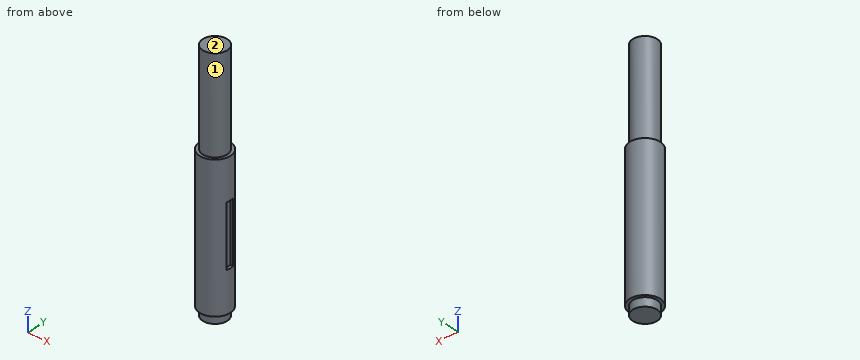
from build123d import *

# Parameters (mm, degrees)
SKETCH1_R           = 12.5
BOSS_EXTRUDE1_DEPTH = 116
SKETCH2_R           = 10
BOSS_EXTRUDE2_DEPTH = 7
BOSS_EXTRUDE3_START = 7
SKETCH3_R           = 10
BOSS_EXTRUDE3_DEPTH = 7
SKETCH4_W           = 50
SKETCH4_H           = 6.35
CUT_EXTRUDE1_DEPTH  = 2.38125
SKETCH6_R           = 10
BOSS_EXTRUDE4_DEPTH = 70


with BuildPart() as part:
    # Sketch1 → Boss-Extrude1 (new body)
    with BuildSketch(Plane.XY):
        with Locations(Location((0, 0, 0), (0, 0, 180))):
            Circle(SKETCH1_R)
    extrude(amount=BOSS_EXTRUDE1_DEPTH)

    # Sketch2 → Boss-Extrude2 (add)
    with BuildSketch(Plane.XY.offset(116)):
        Circle(SKETCH2_R)
    extrude(amount=BOSS_EXTRUDE2_DEPTH)

    # Sketch3 → Boss-Extrude3 (add)
    with BuildSketch(Plane(origin=(0, 0, 0), x_dir=(-1, 0, 0), z_dir=(0, 0, -1)).offset(BOSS_EXTRUDE3_START)):
        with Locations(Location((0, 0, 0), (0, 0, 180))):
            Circle(SKETCH3_R)
    extrude(amount=-BOSS_EXTRUDE3_DEPTH)

    # Sketch4 → Cut-Extrude1 (cut)
    with BuildSketch(Plane(origin=(12.5, 0, 0), x_dir=(0, 0, -1), z_dir=(1, 0, 0))):
        with Locations((-58, 0)):
            Rectangle(SKETCH4_W, SKETCH4_H)
    extrude(amount=-CUT_EXTRUDE1_DEPTH, mode=Mode.SUBTRACT)

    # Sketch6 → Boss-Extrude4 (add)
    with BuildSketch(Plane.XY.offset(123)):
        Circle(SKETCH6_R)
    extrude(amount=BOSS_EXTRUDE4_DEPTH)


solid = part.part
Verification items for the finished model (mm, model axes). Face numbers are marked on the shaded views. A direction names the side the tool comes from. Round coordinates to 2 decimals unless told otherwise and drop trailing zeros. Loops run counter-clockwise (first coordinate to the right, second up) from the corner with the lowest first, then second, coordinate; pieces in that order, holes last. Notation, with made-up numbers: (81, 35.25) - (105, 35.25) arc R4 cw to (105, 41.25) - close; hole circle Ø11 at (25, -6.75). An arc over 180 degrees is marked (long way). Use a Markdown table: item, result. Add a question column.
1. Section check A-A, the plane y = 0. Record the boundary of the cut face in (x, z).
2. Thickness scan on probe 1 along X at (y, z) = (-7.5, 8); probe 2 along Z at (x, y) = (-4.5, -9); probe 3 along Y at (x, z) = (0, 66.5). Record the ranges inside material, lowest first. Write a range as [from, to].
3. Gauge pin test, flat ends, axial feed: pin 1 (8 mm diameter, centred on y = 4.5, z = 102, fed in from -X); pin 2 (3 mm diameter, centred on y = -1, z = 55.5, fed in from +X); pin 3 (2 mm diameter, centred on y = -2.5, z = 31, fed in from +X). Record the tip position at first contact, or that the pin passes through.
4. Section check C-C, the plane z = 152.5. Record the boundary of the cut face in (x, y).
5. Section check D-D, the plane z = 78.5. Record the boundary of the cut face in (x, y) (3 decimals).
6. Access from +Z, -Z, +X, -X, +Y, -Y to the whole of each face (thin tool, end or side, straight path). Record for the marked faces 1 and 2.
7. Section check B-B, the plane x = 0. Record the boundary of the cut face in (y, z), plus the area to 3 significant figures.
Checks:
| question | item | result |
|---|---|---|
| 1 | outline | (-12.5, 0) - (-10, 0) - (-10, -7) - (10, -7) - (10, 0) - (12.5, 0) - (12.5, 33) - (10.12, 33) - (10.12, 83) - (12.5, 83) - (12.5, 116) - (10, 116) - (10, 193) - (-10, 193) - (-10, 116) - (-12.5, 116) - close |
| 2 | probe 1 | x = [-10, 10] |
| 2 | probe 2 | z = [0, 116] |
| 2 | probe 3 | y = [-12.5, 12.5] |
| 3 | pin 1 | stops at x = -12.49 |
| 3 | pin 2 | stops at x = 10.12 |
| 3 | pin 3 | stops at x = 12.41 |
| 4 | outline | circle Ø20 at (0, 0) |
| 5 | outline | (10.119, -3.175) - (10.119, 3.175) - (12.09, 3.175) arc R12.5 ccw (long way) to (12.09, -3.175) - close |
| 6 | face 1 | +Z |
| 6 | face 2 | +Z, +X, -X, +Y, -Y |
| 7 | outline | (-12.5, 0) - (-10, 0) - (-10, -7) - (10, -7) - (10, 0) - (12.5, 0) - (12.5, 116) - (10, 116) - (10, 193) - (-10, 193) - (-10, 116) - (-12.5, 116) - close |
| 7 | area | 4,580 mm^2 |
